```python
from build123d import *

# Parameters (mm, degrees)
BOSS_EXTRUDE1_DEPTH    = 34.29
SKETCH2_W              = 4.699
SKETCH2_H              = 1.905
CUT_EXTRUDE1_DEPTH     = 60.774381845
SKETCH3_W              = 3.175
SKETCH3_H              = 4.572
CUT_EXTRUDE2_DEPTH     = 9.779
CUT_EXTRUDE3_DEPTH     = 70.085665402
CUT_EXTRUDE4_START     = -26.543
CUT_EXTRUDE4_OUTLINE_W = 7.62
CUT_EXTRUDE4_OUTLINE_H = 4.7625
CUT_EXTRUDE4_DEPTH     = 26.543
FILLET4_R              = 1.5875


# Read off the part's stored shape, not the designer's step: Cut-Extrude4
with BuildPart() as part:
    # Sketch1 → Boss-Extrude1 (new body)
    with BuildSketch(Plane.XY):
        Polygon((9.398, 6.35), (9.398, -6.35), (9.398, -7.774459459), (11.938, -8.255), (11.938, -6.35), (51.689, -6.35), (51.689, -8.255), (54.483, -8.255), (54.483, -3.4925), (57.658, -3.4925), (57.658, 3.4925), (54.483, 3.4925), (54.483, 8.255), (51.689, 8.255), (51.689, 6.35), (11.938, 6.35), (11.938, 8.255), (9.398, 7.774459459), align=None)
    extrude(amount=-BOSS_EXTRUDE1_DEPTH)

    # Sketch2 → Cut-Extrude1 (cut, through all)
    with BuildSketch(Plane.ZY.offset(-9.398)):
        with Locations((-2.3495, 7.3025)):
            Rectangle(SKETCH2_W, SKETCH2_H)
        Polygon((-4.699, -8.255), (-4.699, -1.27), (0, 0.889), (0, -8.255), align=None)
    extrude(amount=-CUT_EXTRUDE1_DEPTH, mode=Mode.SUBTRACT)

    # Sketch3 → Cut-Extrude2 (cut)
    with BuildSketch(Plane.XY):
        with Locations((36.7665, -0.381)):
            Rectangle(SKETCH3_W, SKETCH3_H)
    extrude(amount=-CUT_EXTRUDE2_DEPTH, mode=Mode.SUBTRACT)

    # Sketch4 → Cut-Extrude3 (cut, through all)
    with BuildSketch(Plane.XZ.offset(8.255)):
        with BuildLine():
            Line((51.689, -34.29), (51.689, -7.747))
            Line((51.689, -7.747), (40.767, -7.747))
            Line((40.767, -7.747), (40.767, -10.668))
            ThreePointArc((40.767, -10.668), (40.320630735, -11.745630735), (39.243, -12.192))
            Line((39.243, -12.192), (34.671, -12.192))
            ThreePointArc((34.671, -12.192), (33.593369265, -11.745630735), (33.147, -10.668))
            Line((33.147, -10.668), (33.147, -7.747))
            Line((33.147, -7.747), (25.4, -7.747))
            Line((25.4, -7.747), (25.4, -16.637))
            Line((25.4, -16.637), (15.875, -16.637))
            Line((15.875, -16.637), (15.875, -7.747))
            Line((15.875, -7.747), (15.748, -7.747))
            ThreePointArc((15.748, -7.747), (13.053923164, -8.862923164), (11.938, -11.557))
            Line((11.938, -11.557), (11.938, -34.29))
            Line((11.938, -34.29), (51.689, -34.29))
        make_face()
        with BuildLine():
            Line((35.179, -7.747), (38.354, -7.747))
            Line((38.354, -7.747), (38.354, -9.525))
            ThreePointArc((38.354, -9.525), (38.130815367, -10.063815367), (37.592, -10.287))
            Line((37.592, -10.287), (35.941, -10.287))
            ThreePointArc((35.941, -10.287), (35.402184633, -10.063815367), (35.179, -9.525))
            Line((35.179, -9.525), (35.179, -7.747))
        make_face()
        Polygon((57.658, -4.699), (54.483, -4.699), (51.562, 0), (57.658, 0), align=None)
        Polygon((6.604, -4.699), (12.319, -4.699), (24.892, 0), (6.604, 0), align=None)
    extrude(amount=-CUT_EXTRUDE3_DEPTH, mode=Mode.SUBTRACT)

    # Cut-Extrude4 outline → Cut-Extrude4 (cut)
    with BuildSketch(Plane(origin=(0, 0, -34.29), x_dir=(-1, 0, 0), z_dir=(0, 0, -1)).offset(CUT_EXTRUDE4_START)):
        with BuildLine():
            Line((-22.225, -6.35), (-15.875, -6.35))
            Line((-15.875, -6.35), (-15.875, -5.021000706))
            Line((-15.875, -5.021000706), (-11.938, -5.021000706))
            Line((-11.938, -5.021000706), (-9.906, -4.636568273))
            Line((-9.906, -4.636568273), (-9.906, 4.636568273))
            Line((-9.906, 4.636568273), (-11.938, 5.021000706))
            Line((-11.938, 5.021000706), (-15.875, 5.021000706))
            Line((-15.875, 5.021000706), (-15.875, 6.35))
            Line((-15.875, 6.35), (-22.225, 6.35))
            ThreePointArc((-22.225, 6.35), (-15.875, 0), (-22.225, -6.35))
        make_face()
        with Locations((-36.957, -3.96875)):
            Rectangle(CUT_EXTRUDE4_OUTLINE_W, CUT_EXTRUDE4_OUTLINE_H)
        with BuildLine():
            Line((-25.4, 4.7752), (-25.4, -4.7752))
            Line((-25.4, -4.7752), (-22.225, -4.7752))
            ThreePointArc((-22.225, -4.7752), (-17.4498, 0), (-22.225, 4.7752))
            Line((-22.225, 4.7752), (-25.4, 4.7752))
        make_face()
        with Locations((-36.957, 3.96875)):
            Rectangle(CUT_EXTRUDE4_OUTLINE_W, CUT_EXTRUDE4_OUTLINE_H)
        Polygon((-54.181998462, -1.397), (-51.689, -5.715), (-51.689, 5.715), (-54.181998462, 1.397), (-55.753, 1.397), (-55.753, -1.397), align=None)
    extrude(amount=CUT_EXTRUDE4_DEPTH, mode=Mode.SUBTRACT)

    # Fillet4
    fillet4_edges = [part.edges().sort_by_distance(p)[0] for p in [
        (38.227, 6.35, 0),
    ]]
    fillet(fillet4_edges, radius=FILLET4_R)


solid = part.part
```
For this review, take the finished solid that the model builds, in its own axes (mm). A direction names the side the tool comes from. Give positions to 0.01 mm unless a question says otherwise; leave off trailing zeros. Write each loop counter-clockwise with the first axis right and the second up, starting at its lowest first coordinate (ties: lowest second). Pieces come first, ordered by that corner, then holes. Notation, with made-up numbers: M -33.5,79.5 L -13.5,79.5 A14 ccw -13.5,102.5 Z; hole C 63.5,12 d3. An arc over 180 degrees is marked long. One line per item, written item: value.
1) The part is to be moulded in two halves that separate along X. For faces 1 (the flat face through (10.65, -8.01, -19.29)), 2 (the flat face through (37, -2.667, -6)), 3 (the flat face through (54.483, 6, -19)), 4 (the flat face through (53, 7, -4.699)), say which applies: +X half, -X half, draft (parallel to the pull), parting line (faces both ways), or undercut.
Results are:
face 1: -X half
face 2: undercut
face 3: +X half
face 4: draft
2) For line 1 (X direction, y = 7.5, z = -14); line 2 (X direction, y = 0.25, z = -12); line 3 (X direction, y = 1.5, z = -16), list the stretches that pass through material, from the lowest coordinate up. Write a range as from..to.
Results are:
line 1: x = 9.4..11.94, 51.69..54.48
line 2: x = 9.4..9.91, 15.88..17.46, 33.93..39.98, 55.75..57.66
line 3: x = 9.4..9.91, 16.05..17.69, 54.12..57.66
3) For faces 5 (the flat face through (54.483, -6, -19)), 6 (the cylindrical face through (40.332, -0.022, -11.734)), 7 (the flat face through (13, 0, -7.747)), list the 3-axis set-ups (+Z, -Z, +X, -X, +Y, -Y) from which the entire face can be reached by the end or side of a thin tool; tool diameter is ignored.
Results are:
face 5: +Z, -Z, +X, -Y
face 6: -Z, +Y, -Y
face 7: -Z
4) Take a section at A-A, the plane z = -22. Write out the cut boundary in (x, y) (1 decimal).
Results are:
outline: M 9.4,-7.8 L 11.9,-8.3 L 11.9,-5 L 9.9,-4.6 L 9.9,4.6 L 11.9,5 L 11.9,8.3 L 9.4,7.8 Z; M 51.7,-8.3 L 54.5,-8.3 L 54.5,-3.5 L 57.7,-3.5 L 57.7,3.5 L 54.5,3.5 L 54.5,8.3 L 51.7,8.3 L 51.7,5.7 L 54.2,1.4 L 55.8,1.4 L 55.8,-1.4 L 54.2,-1.4 L 51.7,-5.7 Z
5) For P1, Ø3.5, axis at x = 36.5, y = 0, coming from the -Z side; P2, Ø1, axis at x = 48, y = -2.5, coming from the +Z side; P3, Ø4, axis at x = 29, z = -14, coming from the +Y side; P4, Ø7.5, axis at x = 33.5, z = -7.5, coming from the +Y side, all flat-tipped, find the tip position at first contact; note any pin that passes through.
Results are:
P1: stops at z = -12.19
P2: stops at z = -4.7
P3: passes through
P4: stops at y = 6.35
